Here's how the part is built. I have some questions about the finished solid (model axes, mm). A direction names the side the tool comes from. Coordinates: 2 decimals unless noted, no trailing zeros. Write each loop counter-clockwise with the first axis right and the second up, starting at its lowest first coordinate (ties: lowest second). Pieces come first, ordered by that corner, then holes.
from build123d import *


with BuildPart() as part:
    # 草图1 → 旋转1 (revolve)
    with BuildSketch(Plane.XY):
        with BuildLine():
            Line((-70.913736012, 0), (-70.913736012, 3.5))
            Line((-70.913736012, 3.5), (-70.413736012, 4))
            Line((-70.413736012, 4), (-68.413986014, 4))
            Line((-68.413986014, 4), (-68.413986014, 3.8))
            Line((-68.413986014, 3.8), (-67.513986014, 3.8))
            Line((-67.513986014, 3.8), (-67.513986014, 4))
            Line((-67.513986014, 4), (-52.513986014, 4))
            Line((-52.513986014, 4), (-52.513986014, 3.6))
            Line((-52.513986014, 3.6), (-50.913986014, 3.6))
            Line((-50.913986014, 3.6), (-50.913986014, 4.1))
            Line((-50.913986014, 4.1), (-50.913986014, 5))
            Line((-50.913986014, 5), (-46.913986014, 5))
            ThreePointArc((-46.913986014, 5), (-46.772564658, 5.058578644), (-46.713986014, 5.2))
            Line((-46.713986014, 5.2), (-46.713986014, 6))
            Line((-46.713986014, 6), (-31.913986014, 6))
            ThreePointArc((-31.913986014, 6), (-31.772564658, 6.058578644), (-31.713986014, 6.2))
            Line((-31.713986014, 6.2), (-31.713986014, 7))
            Line((-31.713986014, 7), (-29.713986014, 7))
            Line((-29.713986014, 7), (-29.713986014, 0))
            Line((-29.713986014, 0), (-70.913736012, 0))
        make_face()
    revolve(axis=Axis((-99.953379953, 0, 0), (1, 0, 0)))


solid = part.part
1. Thinking about a two-plate mould opening in X: for faces 4 (the face through (-51.703, 3.434, 1.081)), 5 (the face through (-70.914, 0, 0)), 6 (the face through (-39, -6, 0)), which applies, pulls with the +X half, pulls with the -X half, needs draft (parallel to the pull), parting line crosses it, or undercut?
2. If I drill on line 1 (X direction, y = 4, z = 2.5); line 2 (X direction, y = -2.75, z = 2.75); line 3 (X direction, y = -2.5, z = -5.75), over which ranges is the centre line in solid material (lowest first)?
3. I want a section at C-C (x = -67). List the corners of the cut face in (y, z) for me.
4. On a 3-axis mill with a long thin cutter (end or side, diameter ignored), from which of +Z, -Z, +X, -X, +Y, -Y can I reach the whole of each face in a straight line? I mean faces 1 (the face through (-46.714, 2, 5)), 2 (the face through (-29.714, 0, 0)), 3 (the face through (-50.914, -3.3, -2.2)). Say none if no direction works.
5. I want a section at D-D (x = -33.5). List the corners of the cut face in (y, z) for me, then the cut area to 3 significant figures.
6. For pin 1 Ø8 at (x, z) = (-59.5, -1.5) entering from +Y; pin 2 Ø8 at (x, z) = (-45, -1.5) entering from -Y; pin 3 Ø8 at (x, y) = (-61, 2) entering from -Z, each with a flat end and sliding along its axis, tell me the tip position at first contact or that it passes through.
Response values:
1. face 4: undercut
1. face 5: pulls with the -X half
1. face 6: needs draft
2. line 1: x = -50.91 to -29.71
2. line 2: x = -70.52 to -68.41, -67.51 to -52.51, -50.91 to -29.71
2. line 3: x = -31.71 to -29.71
3. outline: circle Ø8 at (0, 0)
4. face 1: -X
4. face 2: +Z, -Z, +X, +Y, -Y
4. face 3: none
5. outline: circle Ø12 at (0, 0)
5. area: 113 mm2
6. pin 1: stops at y = 4
6. pin 2: stops at y = -6
6. pin 3: stops at z = -4
